The listing builds one solid part. Answer for the finished solid, in the listing's coordinates (mm). Coordinates: 2 decimals unless noted, no trailing zeros. Loops run counter-clockwise (first coordinate to the right, second up) from the corner with the lowest first, then second, coordinate; pieces in that order, holes last. Notation, with made-up numbers: (-14, 28) - (14, 28) arc R24 ccw to (14, 41) - close; hole circle Ø9 at (63, -15.75). An arc over 180 degrees is marked (long way). Return JSON: item names as keys, results as strings. Group by question number.
1. Find the intervals of material crossed by line 1 along X through (y, z) = (-0.75, 93); line 2 along Z through (x, y) = (-4.25, -0.5); line 3 along Z through (x, y) = (-2.5, 4.5), in increasing order.
2. Section C-C (y = 0) is taken. Write down the section's boundary in (x, z) (3 decimals), and give its area (3 significant figures).
3. Each of these flat-tipped pins is pushed along its axis until it touches: P1, Ø10, axis at x = 3, y = -6, coming from the -Z side; P2, Ø1, axis at y = 2.5, z = 32.5, coming from the -X side; P3, Ø5, axis at x = 0, y = -5, coming from the +Z side. Where does it stop, or does it pass through?
4. Section A-A (z = 53) is taken. Write down the section's boundary in (x, y) (3 decimals), and give its area (3 significant figures).
5. Section B-B (x = 0) is taken. Write down the section's boundary in (y, z) (1 decimal), and give its area (3 significant figures).
Autodesk Inventor part; units mm, degrees
ref_plane "Start Plane" through (0, 0, -14.9225) normal (0, 0, 1) x (1, 0, 0)
ref_plane "End Plane" through (0, 0, 172.9966) normal (0, 0, 1) x (1, 0, 0)
ref_plane "Work Plane4" through (0, 9.525, 172.9966) normal (0, -0.1054, 0.9944) x (1, 0, 0)
ref_plane "Start Plane" through (0, 0, -14.9225) normal (0, 0, 1) x (1, 0, 0)
ref_plane "End Plane" through (0, 0, 172.9966) normal (0, 0, 1) x (1, 0, 0)
sketch "Sketch" plane through (0, 0, 0) normal (0, 0, 1) x (1, 0, 0)
  circle A0 centre (0, 0) radius 9.525
  dimension "d0" = 19.05
extrude "Body" add sketch "Sketch" along normal up to surface (187.9191 mm away) from surface at -14.9225
sketch "Sketch2" plane through (0, 0, 0) normal (0, 0, 1) x (1, 0, 0)
  line L0 (0, 0) -> (10, 0)
ref_plane "Work Plane3" through (0, 0, 0) normal (0, -1, 0) x (1, 0, 0)
ref_plane "Work Plane4" through (0, 9.525, 172.9966) normal (0, -0.1054, 0.9944) x (1, 0, 0)
split "Split1" plane through (0, 9.525, 172.9966) removes the side toward (0, -0.1054, 0.9944)
ref_plane "Work Plane5" through (0, 9.525, -14.9225) normal (0, -0.8429, -0.538) x (1, 0, 0)
split "Split2" plane through (0, 9.525, -14.9225) removes the side toward (0, -0.8429, -0.538)
sketch "Sketch3" plane through (0, 0, 0) normal (0, -1, 0) x (1, 0, 0)
  line L0 (-2, -14.9225) -> (12, -14.9225)
  line L1 (-2, 172.9966) -> (12, 172.9966)
  dimension "d7" = 187.9191
equation "\"d0\" = Diam"
equation "\"d1\" = G_L"
equation "\"Diam\" = 19.05"
equation "\"G_L\" = d7"
equation "\"G_OFFSET_START\" = 14.92247"
equation "\"G_OFFSET_END\" = 1.00953"
equation "\"d4\" = -G_OFFSET_START"
equation "\"d5\" = G_OFFSET_END + B_L"
equation "\"B_L\" = 171.98707"
properties part number "ANSI/AISC Rolled Steel - 3/4-7.398, RB" material "Steel, Mild"
The answers:
{
 "1": {"line 1": "x = -9.5 to 9.5", "line 2": "z = 0.78 to 171.93", "line 3": "z = -7.05 to 172.46"},
 "2": {"outline": "(-9.525, 0.001) - (9.525, 0.001) - (9.525, 171.987) - (-9.525, 171.987) - close", "area": "3,280 mm2"},
 "3": {"P1": "stops at z = 1.57", "P2": "stops at x = -9.31", "P3": "stops at z = 171.72"},
 "4": {"outline": "circle Ø19.05 at (0, 0)", "area": "285 mm2"},
 "5": {"outline": "(-9.5, 14.9) - (9.5, -14.9) - (9.5, 173) - (-9.5, 171) - close", "area": "3,280 mm2"}
}
